```python
from build123d import *

# Parameters (mm, degrees)
F1_DEPTH = 41.275
F3_DEPTH = 67.31
F4_SIZE  = 2


with BuildPart() as f1:
    # F0 (on Front) → F1 (new body)
    with BuildSketch(Plane.XZ):
        with BuildLine():
            Line((0, 42.709876), (0, 0))
            Line((0, 0), (56.735039, 0))
            Line((56.735039, 0), (56.735039, 42.709876))
            ThreePointArc((56.735039, 42.709876), (28.367519, 71.077395), (0, 42.709876))
        make_face()
    extrude(amount=F1_DEPTH)

    # F2 (on face) → F3 (cut)
    with BuildSketch(Plane.YZ.offset(56.735039)):
        with BuildLine():
            ThreePointArc((-25.487708, 33.117347), (-27.786179, 10.816629), (-7.998581, 21.354938))
            ThreePointArc((-7.998581, 21.354938), (-10.42517, 28.821331), (-16.77764, 33.434517))
            Line((-16.77764, 33.434517), (-16.77764, 30.423621))
            Line((-16.77764, 30.423621), (-25.487708, 30.423621))
            Line((-25.487708, 30.423621), (-25.487708, 33.117347))
        make_face()
    extrude(amount=-F3_DEPTH, mode=Mode.SUBTRACT)

    # F4
    f4_edges = [f1.edges().sort_by_distance(p)[0] for p in [
        (28.367519, -41.275, 71.077395),
        (56.735039, 0, 21.354938),
    ]]
    chamfer(f4_edges, length=F4_SIZE)


solid = f1.part
```
The model under review builds one solid part; all positions refer to its coordinate system, in mm. A direction names the side the tool comes from. Round coordinates to 2 decimals unless told otherwise and drop trailing zeros. Write each loop counter-clockwise with the first axis right and the second up, starting at its lowest first coordinate (ties: lowest second). Pieces come first, ordered by that corner, then holes. Notation, with made-up numbers: (32.5, 13.5) - (53.5, 13.5) arc R32 ccw to (53.5, 49.5) - close; hole circle Ø3 at (60.25, 52). An arc over 180 degrees is marked (long way). Answer as CSV lines item,"result". Start each with the question number.
(1) To check wall thickness, follow line 1 (Z direction, x = 11, y = -14); line 2 (Y direction, x = 42, z = 24) (3 decimals); line 3 (Z direction, x = 43, y = -29.5). State the ranges of each line that lie inside material, in increasing order.
(2) We need section A-A on y = -30. State the section outline as (x, z) points, plus the area to 3 significant figures.
(3) For faces 4 (the flat face through (28, -41.275, 35)), 5 (the flat face through (29, -21, 30.424)), list the 3-axis set-ups (+Z, -Z, +X, -X, +Y, -Y) from which the entire face can be reached by the end or side of a thin tool; tool diameter is ignored.
(4) We need section C-C on y = -14. State the section outline as (x, z) points, plus the area to 3 significant figures.
(5) We need section B-B on y = -4. State the section outline as (x, z) points.
(6) Draft analysis for pull direction Z (two halves, no side actions). For faces 1 (the conical face through (28.954, -40.956, 69.39)), 2 (the flat face through (1, -1, 22)), 3 (the flat face through (29, -25.488, 32)), state which applies: pulls with the +Z half, pulls with the -Z half, needs draft (parallel to the pull), parting line crosses it, or undercut.
Worked answers:
1,line 1,"0 to 10.57, 32.14 to 65.14"
1,line 2,"-41.275 to -33.12, -8.277 to 0"
1,line 3,"0 to 12.2, 30.51 to 67.01"
2,outline,"(0, 0) - (56.74, 0) - (56.74, 12.71) - (0, 12.71) - close; (0, 30) - (56.74, 30) - (56.74, 42.71) arc R28.37 ccw to (0, 42.71) - close"
2,area,"2,710 mm²"
3,face 4,"+Z, -Z, +X, -X, -Y"
3,face 5,"+X, -X"
4,outline,"(0, 0) - (56.74, 0) - (56.74, 10.57) - (0, 10.57) - close; (0, 32.14) - (56.74, 32.14) - (56.74, 42.71) arc R28.37 ccw to (0, 42.71) - close"
4,area,"2,460 mm²"
5,outline,"(0, 0) - (56.74, 0) - (56.74, 42.71) arc R28.37 ccw to (0, 42.71) - close"
6,face 1,"pulls with the +Z half"
6,face 2,"needs draft"
6,face 3,"undercut"
